Here's how the part is built. I have some questions about the finished solid (model axes, mm). Face numbers are marked on the shaded views. A direction names the side the tool comes from. Give positions to 0.01 mm unless a question says otherwise; leave off trailing zeros. Loops run counter-clockwise (first coordinate to the right, second up) from the corner with the lowest first, then second, coordinate; pieces in that order, holes last. Notation, with made-up numbers: (61, 12.25) - (118, 12.25) arc R29 cw to (118, 37.25) - close; hole circle Ø8 at (16.25, -11.5). An arc over 180 degrees is marked (long way). Use a Markdown table: item, result.
from build123d import *

# Parameters (mm, degrees)
ESQUISSE1_W             = 17
ESQUISSE1_H             = 26
BOSS_EXTRU_1_DEPTH      = 3
ESQUISSE3_W             = 4
ESQUISSE3_H             = 26
BOSS_EXTRU_2_DEPTH      = 38
ESQUISSE4_R             = 1.5
ENL_V_MAT_EXTRU_2_DEPTH = 4
ESQUISSE5_R             = 1.5
ENL_V_MAT_EXTRU_3_DEPTH = 4
ESQUISSE6_W             = 3
ESQUISSE6_H             = 26
BOSS_EXTRU_3_DEPTH      = 13
ESQUISSE8_R             = 5.25
ENL_V_MAT_EXTRU_4_DEPTH = 2
ENL_V_START             = -2
ESQUISSE9_R             = 5.25
ENL_V_MAT_EXTRU_5_DEPTH = 2
ESQUISSE10_W            = 17
ESQUISSE10_H            = 4
BOSS_EXTRU_5_DEPTH      = 0.5
ESQUISSE11_W            = 17
ESQUISSE11_H            = 4.5
ENL_V_MAT_EXTRU_6_DEPTH = 0.5


with BuildPart() as part:
    # Esquisse1 → Boss.-Extru.1 (new body)
    with BuildSketch(Plane.XY):
        with Locations((8.5, 13)):
            Rectangle(ESQUISSE1_W, ESQUISSE1_H)
    extrude(amount=BOSS_EXTRU_1_DEPTH)

    # Esquisse3 → Boss.-Extru.2 (add)
    with BuildSketch(Plane(origin=(0, 0, 0), x_dir=(-1, 0, 0), z_dir=(0, 0, -1))):
        with Locations((-2, 13)):
            Rectangle(ESQUISSE3_W, ESQUISSE3_H)
    extrude(amount=BOSS_EXTRU_2_DEPTH)

    # Esquisse4 → Enlèv. mat.-Extru.2 (cut)
    with BuildSketch(Plane.ZY):
        with Locations((-8.5, 20)):
            Circle(ESQUISSE4_R)
        with Locations((-8.5, 6)):
            Circle(ESQUISSE4_R)
    extrude(amount=-ENL_V_MAT_EXTRU_2_DEPTH, mode=Mode.SUBTRACT)

    # Esquisse5 → Enlèv. mat.-Extru.3 (cut)
    with BuildSketch(Plane.ZY):
        with Locations((-26.5, 19.999545392)):
            Circle(ESQUISSE5_R)
        with Locations((-26.5, 6)):
            Circle(ESQUISSE5_R)
    extrude(amount=-ENL_V_MAT_EXTRU_3_DEPTH, mode=Mode.SUBTRACT)

    # Esquisse6 → Boss.-Extru.3 (add)
    with BuildSketch(Plane(origin=(4, 0, 0), x_dir=(0, 0, -1), z_dir=(1, 0, 0))):
        with Locations((36.5, 13)):
            Rectangle(ESQUISSE6_W, ESQUISSE6_H)
    extrude(amount=BOSS_EXTRU_3_DEPTH)

    # Esquisse8 → Enlèv. mat.-Extru.4 (cut)
    with BuildSketch(Plane(origin=(0, 0, 0), x_dir=(-1, 0, 0), z_dir=(0, 0, -1))):
        with Locations((-10, 7)):
            Circle(ESQUISSE8_R)
        with Locations((-10, 19)):
            Circle(ESQUISSE8_R)
    extrude(amount=-ENL_V_MAT_EXTRU_4_DEPTH, mode=Mode.SUBTRACT)

    # Esquisse9 → Enlèv. mat.-Extru.5 (cut)
    with BuildSketch(Plane.XY.offset(-35).offset(ENL_V_START)):
        with Locations(Location((10, 19, 0), (0, 0, 180))):
            Circle(ESQUISSE9_R)
        with Locations(Location((10, 7, 0), (0, 0, 180))):
            Circle(ESQUISSE9_R)
    extrude(amount=ENL_V_MAT_EXTRU_5_DEPTH, mode=Mode.SUBTRACT)

    # Esquisse10 → Boss.-Extru.5 (add)
    with BuildSketch(Plane.XY.offset(3)):
        with Locations((8.5, 13)):
            Rectangle(ESQUISSE10_W, ESQUISSE10_H)
    extrude(amount=BOSS_EXTRU_5_DEPTH)

    # Esquisse11 → Enlèv. mat.-Extru.6 (cut)
    with BuildSketch(Plane(origin=(0, 0, -38), x_dir=(-1, 0, 0), z_dir=(0, 0, -1))):
        with Locations((-8.5, 13)):
            Rectangle(ESQUISSE11_W, ESQUISSE11_H)
    extrude(amount=-ENL_V_MAT_EXTRU_6_DEPTH, mode=Mode.SUBTRACT)


solid = part.part
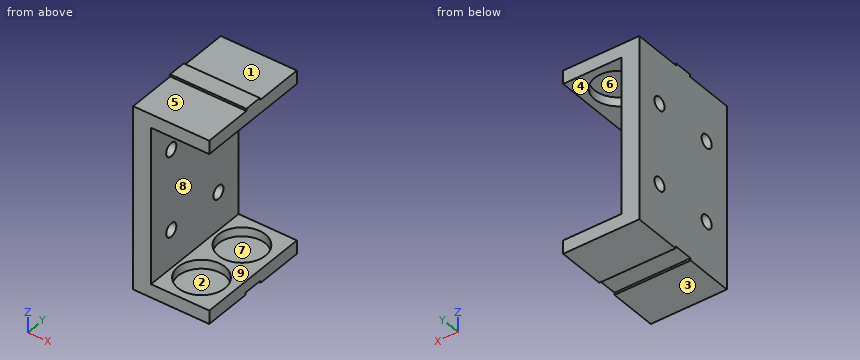
(1) We'd pull the mould along X, two halves only. Please class the marked faces 6, 7, 8 and 9: pulls with the +X half, pulls with the -X half, needs draft (parallel to the pull), parting line crosses it, or undercut.
A:
| item | result |
|---|---|
| face 6 | undercut |
| face 7 | undercut |
| face 8 | pulls with the +X half |
| face 9 | needs draft |
(2) If I drill on line 1 (Y direction, x = 3.5, z = -26.5); line 2 (Z direction, x = 6.75, y = 8); line 3 (Y direction, x = 10, z = 1.25), over which ranges is the centre line in solid material (lowest first)?
A:
| item | result |
|---|---|
| line 1 | 0 to 4.5, 7.5 to 18.5, 21.5 to 26 |
| line 2 | -38 to -37, 2 to 3 |
| line 3 | 0 to 1.75, 12.25 to 13.75, 24.25 to 26 |
(3) Suppose I cut it at D-D on z = 0.5. Write out the boundary of the cut face in (x, y), plus the area to 3 significant figures.
A:
| item | result |
|---|---|
| outline | (0, 0) - (17, 0) - (17, 26) - (0, 26) - close; hole circle Ø10.5 at (10, 7); hole circle Ø10.5 at (10, 19) |
| area | 269 mm2 |
(4) Will these pins go through, and if not, where does the flat tip stop? pin 1 (5 mm diameter, centred on y = 6, z = -26.5, fed in from +X); pin 2 (1.8 mm diameter, centred on y = 20, z = -26.5, fed in from -X); pin 3 (1 mm diameter, centred on x = 14.5, y = 11.5, fed in from -Z); pin 4 (9 mm diameter, centred on x = 8, y = 3.5, fed in from +Z).
A:
| item | result |
|---|---|
| pin 1 | x = 4 |
| pin 2 | through |
| pin 3 | z = -37.5 |
| pin 4 | z = 3 |
(5) On a 3-axis mill with a long thin cutter (end or side, diameter ignored), from which of +Z, -Z, +X, -X, +Y, -Y can I reach the whole of each face in a straight line? I mean the marked faces 1, 2, 3, 4 and 5. Say none if no direction works.
A:
| item | result |
|---|---|
| face 1 | +Z, +X, -X, +Y |
| face 2 | none |
| face 3 | -Z, +X, -X, +Y, -Y |
| face 4 | +X, +Y, -Y |
| face 5 | +Z, +X, -X, -Y |
(6) Suppose I cut it at B-B on z = -26.5. Write out the boundary of the cut face in (x, y).
A:
| item | result |
|---|---|
| outline | (0, 0) - (4, 0) - (4, 4.5) - (0, 4.5) - close; (0, 7.5) - (4, 7.5) - (4, 18.5) - (0, 18.5) - close; (0, 21.5) - (4, 21.5) - (4, 26) - (0, 26) - close |
(7) Suppose I cut it at C-C on y = 19. Write out the boundary of the cut face in (x, z).
A:
| item | result |
|---|---|
| outline | (0, -38) - (17, -38) - (17, -35) - (15.25, -35) - (15.25, -37) - (4.75, -37) - (4.75, -35) - (4, -35) - (4, -27.62) - (0, -27.62) - close; (0, -25.38) - (4, -25.38) - (4, -9.62) - (0, -9.62) - close; (0, -7.38) - (4, -7.38) - (4, 0) - (4.75, 0) - (4.75, 2) - (15.25, 2) - (15.25, 0) - (17, 0) - (17, 3) - (0, 3) - close |
